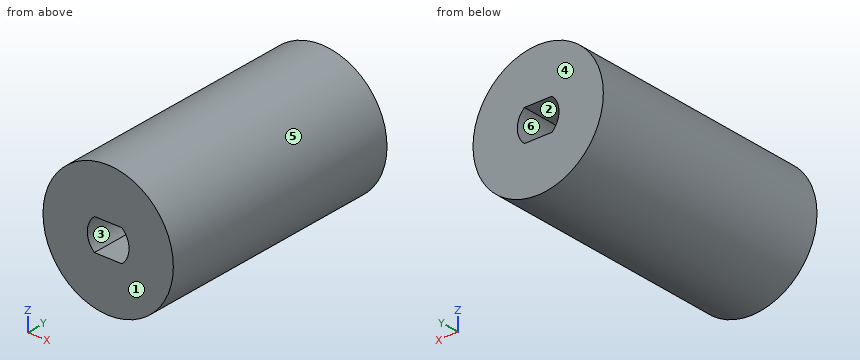
```python
from build123d import *

# Parameters (mm, degrees)
CROQUIS1_R              = 12.5
SALIENTE_EXTRUIR1_DEPTH = 48
CORTAR_EXTRUIR1_DEPTH   = 15
CORTAR_EXTRUIR2_START   = 33
CORTAR_EXTRUIR2_DEPTH   = 15


with BuildPart() as part:
    # Croquis1 → Saliente-Extruir1 (new body)
    with BuildSketch(Plane(origin=(0, 0, 0), x_dir=(1, 0, 0), z_dir=(0, 1, 0))):
        with Locations(Location((0, 0, 0), (0, 0, 270))):
            Circle(CROQUIS1_R)
    extrude(amount=SALIENTE_EXTRUIR1_DEPTH)

    # Croquis2 → Cortar-Extruir1 (cut)
    with BuildSketch(Plane(origin=(0, 0, 0), x_dir=(1, 0, 0), z_dir=(0, 1, 0))):
        with BuildLine():
            Line((-2.645751311, -3), (2.645751311, -3))
            ThreePointArc((2.645751311, -3), (4, 0), (2.645751311, 3))
            Line((2.645751311, 3), (-2.645751311, 3))
            ThreePointArc((-2.645751311, 3), (-4, 0), (-2.645751311, -3))
        make_face()
    extrude(amount=CORTAR_EXTRUIR1_DEPTH, mode=Mode.SUBTRACT)

    # Croquis2_2 → Cortar-Extruir2 (cut)
    with BuildSketch(Plane(origin=(0, 0, 0), x_dir=(1, 0, 0), z_dir=(0, 1, 0)).offset(CORTAR_EXTRUIR2_START)):
        with BuildLine():
            Line((-2.645751311, -3), (2.645751311, -3))
            ThreePointArc((2.645751311, -3), (4, 0), (2.645751311, 3))
            Line((2.645751311, 3), (-2.645751311, 3))
            ThreePointArc((-2.645751311, 3), (-4, 0), (-2.645751311, -3))
        make_face()
    extrude(amount=CORTAR_EXTRUIR2_DEPTH, mode=Mode.SUBTRACT)


solid = part.part
```
Part model, mm, in its own coordinate system. Face numbers are marked on the shaded views. A direction names the side the tool comes from. Round coordinates to 2 decimals unless told otherwise and drop trailing zeros. Loops run counter-clockwise (first coordinate to the right, second up) from the corner with the lowest first, then second, coordinate; pieces in that order, holes last.
Item 1: Cut at C-C, the plane z = 0. Give the cut face in (x, y).
Item 2: Drill centre lines: line 1 (X direction, y = 37.5, z = -0.25); line 2 (Y direction, x = -2, z = 2.5); line 3 (X direction, y = 43.5, z = 1.25). Where is each one in solid material? Low to high.
Item 3: Cut at A-A, the plane x = 0. Give the cut face in (y, z), then the cut area to 3 significant figures.
Item 4: Cut at D-D, the plane y = 32. Give the cut face in (x, z), then the cut area to 3 significant figures.
Item 5: 3-axis set-ups, long thin cutter, end or side, ignore diameter. For the marked faces 1, 2 and 3: which of +Z, -Z, +X, -X, +Y, -Y reach the whole face in a straight line?
Item 6: Drop flat-ended pins along their axis: P1, Ø2, axis at x = -8.5, y = 5, coming from the -Z side; P2, Ø12, axis at x = -6.5, y = 28, coming from the -Z side; P3, Ø3, axis at y = 30.5, z = 7.5, coming from the -X side. Give the stop position or say it passes through.
Item 7: Cut at B-B, the plane y = 43.5. Give the cut face in (x, z), then the cut area to 3 significant figures.
Item 8: Mould opens along X. For the marked faces 4, 5 and 6 say: +X half, -X half, draft (parallel to the pull), parting line (faces both ways), or undercut.
A:
1. outline: (-12.5, 0) - (-4, 0) - (-4, 15) - (4, 15) - (4, 0) - (12.5, 0) - (12.5, 48) - (4, 48) - (4, 33) - (-4, 33) - (-4, 48) - (-12.5, 48) - close
2. line 1: x = -12.5 to -3.99, 3.99 to 12.5
2. line 2: y = 15 to 33
2. line 3: x = -12.44 to -3.8, 3.8 to 12.44
3. outline: (0, -12.5) - (48, -12.5) - (48, -3) - (33, -3) - (33, 3) - (48, 3) - (48, 12.5) - (0, 12.5) - (0, 3) - (15, 3) - (15, -3) - (0, -3) - close
3. area: 1,020 mm2
4. outline: circle Ø25 at (0, 0)
4. area: 491 mm2
5. face 1: +Z, -Z, +X, -X, -Y
5. face 2: +Y
5. face 3: -Y
6. P1: stops at z = -10
6. P2: stops at z = -12.49
6. P3: stops at x = -10.97
7. outline: circle Ø25 at (0, 0); hole (-2.65, -3) - (2.65, -3) arc R4 ccw to (2.65, 3) - (-2.65, 3) arc R4 ccw to start
7. area: 448 mm2
8. face 4: draft
8. face 5: parting line
8. face 6: undercut
